Autodesk Inventor part; units mm, degrees
ref_plane "Work Plane1" through (-9.8149, 0, 0) normal (0, 0, -1) x (1, 0, 0)
ref_plane "YZ Plane" through (0, 0, 0) normal (1, 0, 0) x (0, 1, 0)
ref_plane "XZ Plane" through (0, 0, 0) normal (0, 1, 0) x (-1, 0, 0)
sketch "Boceto1" plane through (0, 0, 0) normal (1, 0, 0) x (0, 1, 0)
  line L0 (2.3094, -4) -> (-2.3094, -4)
  line L1 (-2.3094, -4) -> (-4.6188, 0)
  line L2 (-4.6188, 0) -> (-2.3094, 4)
  line L3 (-2.3094, 4) -> (2.3094, 4)
  line L4 (2.3094, 4) -> (4.6188, 0)
  line L5 (4.6188, 0) -> (2.3094, -4)
  point P0 (0, 0)
  point P1 (0, 0)
  dimension "d0" = 9.2376
extrude "Cuerpo" add sketch "Boceto1" along normal blind 2.7
sketch "Boceto2" plane through (2.7, 0, 0) normal (1, 0, 0) x (0, 0, -1)
  point P0 (0, 0)
hole "Rosca" at (2.7, 0, 0) direction (-1, 0, 0) diameter 4.134 end through all
chamfer "Chaflán2" distance 0.433 angle 30 1 edges at (2.7, 0, 2.067) measured on face at (2.7, 2.8764, -1.7247)
chamfer "Chaflán1" distance 0.433 angle 30 1 edges at (0, 0, 2.067) measured on face at (0, 2.8764, -1.7247)
ref_plane "Work Plane1" through (-9.8149, 0, 0) normal (0, 0, -1) x (1, 0, 0)
equation "\"d0\" = 1.1547 * SW"
equation "\"d1\" = KOH"
equation "\"d12\" = -0.5 * GD1 + 0.5 * NND"
equation "\"d19\" = -0.5 * GD1 + 0.5 * NND"
equation "\"d10\" = -0.5 * GD1 + 0.5 * NND"
equation "\"d18\" = -0.5 * GD1 + 0.5 * NND"
equation "\"NND\" = 5"
equation "\"KOH\" = 2.7"
equation "\"SW\" = 8"
equation "\"GUL\" = 0.541266 * PTC"
equation "\"THREADDIA\" = 5"
equation "\"TOA\" = 30deg"
equation "\"PTC\" = 0.8"
equation "\"E0\" = 1.155 * SW"
equation "\"GAL\" = 0.541266 * PTC"
properties part number "AS 1474 - M5" material "Acero, suave"
Verification items for the finished model (mm, model axes). Coordinates: 2 decimals unless noted, no trailing zeros. Write each loop counter-clockwise with the first axis right and the second up, starting at its lowest first coordinate (ties: lowest second). Pieces come first, ordered by that corner, then holes. Notation, with made-up numbers: M 67,44 L 74,44 A18 ccw 74,64 Z; hole C 44,-3.5 d8. An arc over 180 degrees is marked long. Answer as a JSON object with one key per item and string values. Group by question number.
(1) Cross-section at D-D, the plane y = 2.75. Record the cut outline in (x, z), and give its area (3 significant figures).
(2) Cross-section at C-C, the plane z = 3.5. Record the cut outline in (x, y).
(3) Cross-section at B-B, the plane x = 1.05. Record the cut outline in (y, z), and give its area (3 significant figures).
(4) Material ranges on line 1 (Z direction, x = 1.55, y = 0); line 2 (Y direction, x = 1.45, z = 1.75); line 3 (Z direction, x = 2.6, y = 1.5), recorded low to high.
(5) Cross-section at A-A, the plane y = 0. Record the cut outline in (x, z), and give its area (3 significant figures).
(6) Gauge pin test, flat end, axial feed: pin 1 (1.5 mm diameter, centred on x = 1, z = -1.5, fed in from -Y). Record the tip position at first contact, or that the pin passes through.
Reply:
{
 "1": {"outline": "M 0,-3.24 L 2.7,-3.24 L 2.7,3.24 L 0,3.24 Z", "area": "17.5 mm²"},
 "2": {"outline": "M 0,-2.6 L 2.7,-2.6 L 2.7,2.6 L 0,2.6 Z"},
 "3": {"outline": "M -4.62,0 L -2.31,-4 L 2.31,-4 L 4.62,0 L 2.31,4 L -2.31,4 Z; hole C 0,0 d4.13", "area": "42.0 mm²"},
 "4": {"line 1": "-4 to -2.07, 2.07 to 4", "line 2": "-3.61 to -1.1, 1.1 to 3.61", "line 3": "-4 to -1.78, 1.78 to 4"},
 "5": {"outline": "M 0,-4 L 2.7,-4 L 2.7,-2.5 L 2.45,-2.07 L 0.25,-2.07 L 0,-2.5 Z; M 0,2.5 L 0.25,2.07 L 2.45,2.07 L 2.7,2.5 L 2.7,4 L 0,4 Z", "area": "10.2 mm²"},
 "6": {"pin 1": "y = -4.19"}
}
